Geometry check sheet. Reference: the model listing, model coordinates, mm. Face numbers are marked on the shaded views. A direction names the side the tool comes from. Coordinates: 2 decimals unless noted, no trailing zeros. Write each loop counter-clockwise with the first axis right and the second up, starting at its lowest first coordinate (ties: lowest second). Pieces come first, ordered by that corner, then holes. Notation, with made-up numbers: M 63.5,-17 L 77.5,-17 A11 cw 77.5,-8 Z; hole C -39,30.25 d8. An arc over 180 degrees is marked long. Write item = value, one per line. Start each with the question number.
```python
from build123d import *

# Parameters (mm, degrees)
F0_R          = 10
F1_DEPTH      = 100
F2_W          = 12
F2_H          = 60
F3_DEPTH      = 100
F3_DEPTH_BACK = 10
F4_W          = 75
F4_H          = 40
F5_DEPTH      = 12
F6_R          = 5
F7_DEPTH      = 100
F8_R          = 5
F9_DEPTH      = 80.001


with BuildPart() as f1:
    # F0 (on Top) → F1 (new body)
    with BuildSketch(Plane.XY):
        Circle(F0_R)
    extrude(amount=F1_DEPTH)

    # F2 (on Front) → F3 (join, two sides)
    with BuildSketch(Plane.XZ) as f3_sk:
        with Locations((0, 50)):
            Rectangle(F2_W, F2_H)
    extrude(amount=F3_DEPTH)
    extrude(f3_sk.sketch, amount=-F3_DEPTH_BACK)

    # F4 (on face) → F5 (cut, through all)
    with BuildSketch(Plane.YZ.offset(6)):
        with Locations((-47.5, 50)):
            Rectangle(F4_W, F4_H)
    extrude(amount=-F5_DEPTH, mode=Mode.SUBTRACT)

    # F6 (on Top) → F7 (cut, through all)
    with BuildSketch(Plane.XY):
        Circle(F6_R)
    extrude(amount=F7_DEPTH, mode=Mode.SUBTRACT)

    # F8 (on face) → F9 (cut, through all)
    with BuildSketch(Plane(origin=(0, 0, 20), x_dir=(1, 0, 0), z_dir=(0, 0, -1))):
        with Locations((0, 92.5)):
            Circle(F8_R)
    extrude(amount=-F9_DEPTH, mode=Mode.SUBTRACT)


solid = f1.part
```
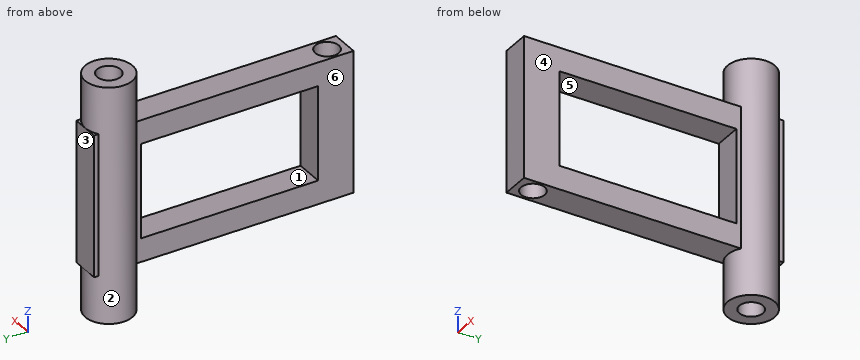
Q1. Cross-section at A-A on z = 44. Enter the section's corners in (x, y).
Q2. Cross-section at D-D on z = 76.5. Enter the section's corners in (x, y), and give its area (3 significant figures).
Q3. Cross-section at C-C on x = 2. Enter the section's corners in (y, z), and give its area (3 significant figures).
Q4. Cross-section at B-B on y = 0. Enter the section's corners in (x, z).
Q5. Draft check along Y on the marked faces 1, 2 and 3. Enter one of: pulls with the +Y half, pulls with the -Y half, needs draft (parallel to the pull), parting line crosses it, or undercut.
Q6. Gauge pin test, flat ends, axial feed: pin 1 (6 mm diameter, centred on x = 0, y = 0, fed in from +Z); pin 2 (1.5 mm diameter, centred on x = -4.5, y = -75, fed in from -Z); pin 3 (3.5 mm diameter, centred on x = -3, y = -56.5, fed in from +Z); pin 4 (0.6 mm diameter, centred on x = -4.5, y = 9, fed in from -Z). Record the tip position at first contact, or that the pin passes through.
Q7. Scan lines: L1, parallel to Y at x = 0, z = 22.5; L2, parallel to Y at x = 0, z = 53.5; L3, parallel to X at y = 0.5, z = 91.5. Record each from-to range of solid material in increasing order.
Q8. Set-up check for the marked faces 4, 5 and 6: record each of +Z, -Z, +X, -X, +Y, -Y from which the full face is reachable in a straight line by a thin tool's end or side.
Values found:
q1.outline = M -6,-100 L 6,-100 L 6,-85 L -6,-85 Z; M -6,-10 L 6,-10 L 6,-8 A10 ccw 6,8 L 6,10 L -6,10 L -6,8 A10 ccw -6,-8 Z; hole C 0,-92.5 d10; hole C 0,0 d10
q2.outline = M -6,-100 L 6,-100 L 6,-8 A10 ccw 6,8 L 6,10 L -6,10 L -6,8 A10 ccw -6,-8 Z; hole C 0,-92.5 d10; hole C 0,0 d10
q2.area = 1,250 mm²
q3.outline = M -100,20 L -97.08,20 L -97.08,80 L -100,80 Z; M -87.92,20 L -9.8,20 L -9.8,0 L -4.58,0 L -4.58,100 L -9.8,100 L -9.8,80 L -87.92,80 Z; M 4.58,0 L 9.8,0 L 9.8,20 L 10,20 L 10,80 L 9.8,80 L 9.8,100 L 4.58,100 Z; hole M -85,30 L -10,30 L -10,70 L -85,70 Z
q3.area = 2,920 mm²
q4.outline = M -10,0 L -5,0 L -5,100 L -10,100 Z; M 5,0 L 10,0 L 10,100 L 5,100 Z
q5.face_1 = undercut
q5.face_2 = parting line crosses it
q5.face_3 = pulls with the +Y half
q6.pin_1 = through
q6.pin_2 = 20
q6.pin_3 = 80
q6.pin_4 = 0
q7.L1 = -100 to -97.5, -87.5 to -5, 5 to 10
q7.L2 = -100 to -97.5, -87.5 to -85, -10 to -5, 5 to 10
q7.L3 = -9.99 to -4.97, 4.97 to 9.99
q8.face_4 = +Z, -Z, +X, -Y
q8.face_5 = +X, -X
q8.face_6 = +Z, -Z, -X, -Y
